Here's how the part is built. I have some questions about the finished solid (model axes, mm). Round coordinates to 2 decimals unless told otherwise and drop trailing zeros. Write each loop counter-clockwise with the first axis right and the second up, starting at its lowest first coordinate (ties: lowest second). Pieces come first, ordered by that corner, then holes. Notation, with made-up numbers: (58, 22) - (102, 22) arc R29 ccw to (102, 56) - close; hole circle Ø3 at (-35.5, 66). An arc over 180 degrees is marked (long way). One line per question, with ' | ' between items. Start each with the question number.
(1) Imagine slicing it at B-B (z = -24). Write out the boundary of the cut face in (x, y), plus the area to 4 significant figures.
(2) Imagine slicing it at A-A (x = -34). Write out the boundary of the cut face in (y, z), plus the area to 3 significant figures.
(3) Will this pin go through, and if not, where does the flat tip stop? pin 1 (3.5 mm diameter, centred on x = -34, z = -35.5, fed in from +Y).
(4) If I drill on L1, parallel to Z at x = 34, y = 0.85; L2, parallel to X at y = 0.25, z = -35, over which ranges is the centre line in solid material (lowest first)?
(5) Imagine slicing it at D-D (y = 0.9). Write out the boundary of the cut face in (x, z), plus the area to 3 significant figures.
(6) Thinking about a two-plate mould opening in X: for faces 1 (the flat face through (1, 0, 1)), 2 (the cylindrical face through (-33.686, 0.74, -34.084)), which applies, pulls with the +X half, pulls with the -X half, needs draft (parallel to the pull), parting line crosses it, or undercut?
(7) Imagine slicing it at C-C (z = -35.5). Write out the boundary of the cut face in (x, y).
Autodesk Inventor part; units mm, degrees
ref_plane "YZ Plane" through (0, 0, 0) normal (1, 0, 0) x (0, 1, 0)
ref_plane "XZ Plane" through (0, 0, 0) normal (0, 1, 0) x (-1, 0, 0)
ref_plane "XY Plane" through (0, 0, 0) normal (0, 0, 1) x (1, 0, 0)
sketch "Sketch1" plane through (0, 0, 0) normal (0, 1, 0) x (-1, 0, 0)
  line L0 (38.5, 38.5) -> (-38.5, 38.5)
  line L1 (-38.5, 38.5) -> (-38.5, -38.5)
  line L2 (-38.5, -38.5) -> (38.5, -38.5)
  line L3 (38.5, -38.5) -> (38.5, 38.5)
  line L4 (38.5, 38.5) -> (-38.5, -38.5) construction
  line L5 (-38.5, 38.5) -> (38.5, -38.5) construction
  point P0 (0, 0)
  dimension "d0" = 77
  dimension "d1" = 77
extrude "Extrusion1" add sketch "Sketch1" along normal blind 1.5
sketch "Sketch2" plane through (0, 0, 0) normal (0, 1, 0) x (-1, 0, 0)
  circle A0 centre (-34, -35.5) radius 1.45
  line L0 (-34, -35.5) -> (-38.5, -35.5) construction
  line L1 (-38.5, 38.5) -> (-38.5, -38.5) construction
  line L2 (-34, -35.5) -> (-34, -38.5) construction
  line L3 (-38.5, -38.5) -> (38.5, -38.5) construction
  line L4 (0, 0) -> (0, -38.5) construction
  line L5 (-38.5, -38.5) -> (38.5, -38.5) construction
  circle A1 centre (34, -35.5) radius 1.45
  line L6 (34, -35.5) -> (38.5, -35.5) construction
  line L7 (34, -35.5) -> (34, -38.5) construction
  dimension "d4" = 2.9
  dimension "d5" = 4.5
  dimension "d6" = 3
extrude "Extrusion2" cut sketch "Sketch2" along normal blind 1.5
sketch "Sketch3" plane through (0, 0, 0) normal (0, 1, 0) x (-1, 0, 0)
  line L0 (18.5, -28.5) -> (28.5, -28.5)
  line L1 (28.5, -28.5) -> (28.5, -18.5)
  line L2 (28.5, -18.5) -> (18.5, -18.5)
  line L3 (18.5, -18.5) -> (18.5, -28.5)
  line L4 (-38.5, -38.5) -> (38.5, -38.5)
  line L5 (38.5, -38.5) -> (38.5, 38.5)
  point P0 (0, 0)
  dimension "d9" = 10
  dimension "d10" = 10
  dimension "d11" = 10
  dimension "d12" = 10
extrude "Extrusion3" cut sketch "Sketch3" along normal blind 10
properties part number "teensy_box_lid"
Check sheet entries:
1) outline: (-38.5, 0) - (-28.5, 0) - (-28.5, 1.5) - (-38.5, 1.5) - close; (-18.5, 0) - (38.5, 0) - (38.5, 1.5) - (-18.5, 1.5) - close | area: 100.5 mm^2
2) outline: (0, -38.5) - (1.5, -38.5) - (1.5, -36.95) - (0, -36.95) - close; (0, -34.05) - (1.5, -34.05) - (1.5, 38.5) - (0, 38.5) - close | area: 111 mm^2
3) pin 1: y = 1.5
4) L1: -38.5 to -36.95, -34.05 to 38.5 | L2: -38.5 to -35.36, -32.64 to 32.64, 35.36 to 38.5
5) outline: (-38.5, -38.5) - (38.5, -38.5) - (38.5, 38.5) - (-38.5, 38.5) - close; hole circle Ø2.9 at (-34, -35.5); hole (-28.5, -28.5) - (-18.5, -28.5) - (-18.5, -18.5) - (-28.5, -18.5) - close; hole circle Ø2.9 at (34, -35.5) | area: 5,820 mm^2
6) face 1: needs draft | face 2: undercut
7) outline: (-38.5, 0) - (-35.45, 0) - (-35.45, 1.5) - (-38.5, 1.5) - close; (-32.55, 0) - (32.55, 0) - (32.55, 1.5) - (-32.55, 1.5) - close; (35.45, 0) - (38.5, 0) - (38.5, 1.5) - (35.45, 1.5) - close
